from build123d import *

# Parameters (mm, degrees)
F0_R           = 90
F3_DEPTH       = 10
F4_D           = 5.5
F4_DEPTH       = 30
F4_TIP         = 1.6523667023
F6_D           = 3.6
F6_CBORE_D     = 6.6
F6_CBORE_DEPTH = 4
F8_D           = 3.6
F8_DEPTH       = 30
F8_TIP         = 1.0815491142
F9_DEPTH       = 5


with BuildPart() as f3:
    # F0 (on Top) → F3 (new body)
    with BuildSketch(Plane.XY):
        Circle(F0_R)
    extrude(amount=F3_DEPTH)

    # F4
    with Locations(Plane(origin=(0, 0, 0), x_dir=(1, 0, 0), z_dir=(0, 0, -1))):
        with Locations((32.5, -56.291651246), (32.5, 56.291651246), (-65, 0), (0, 0)):
            Hole(F4_D / 2, depth=F4_DEPTH)
            with Locations((0, 0, -(F4_DEPTH + F4_TIP / 2))):  # 118° drill point
                Cone(0, F4_D / 2, F4_TIP, mode=Mode.SUBTRACT)

    # F6 (through all)
    with Locations(Plane(origin=(0, 0, 0), x_dir=(1, 0, 0), z_dir=(0, 0, -1))):
        with Locations((14.0151126623, 15.35), (58.0151126623, 15.35), (14.0151126623, -15.35), (58.0151126623, -15.35)):
            CounterBoreHole(F6_D / 2, F6_CBORE_D / 2, F6_CBORE_DEPTH)

    # F8
    with Locations(Plane(origin=(0, 0, 0), x_dir=(1, 0, 0), z_dir=(0, 0, -1))):
        with Locations((-12.8155729771, 59.4439784884), (-20.8155729771, 59.4439784884), (-12.8155729771, 35.4439784884), (-20.8155729771, 35.4439784884), (-49.032068802, -39.4834254403), (-29.032068802, -39.4834254403), (-6.8313475791, -59.4414137304), (8.1686524209, -59.4414137304), (-23.532068802, 0.5165745633), (-54.532068802, 0.5165745597)):
            Hole(F8_D / 2, depth=F8_DEPTH)
            with Locations((0, 0, -(F8_DEPTH + F8_TIP / 2))):  # 118° drill point
                Cone(0, F8_D / 2, F8_TIP, mode=Mode.SUBTRACT)

    # F7 (on face) → F9 (cut)
    with BuildSketch(Plane.XY):
        with BuildLine():
            Line((-54.4565801894, 1.4820002999), (-54.6077416208, 1.4819933337))
            ThreePointArc((-54.6077416208, 1.4819933337), (-56.5317107433, -0.5544177441), (-54.532068802, -2.5165745597))
            ThreePointArc((-54.532068802, -2.5165745597), (-53.1178552397, -1.9307881221), (-52.532068802, -0.5165745597))
            ThreePointArc((-52.532068802, -0.5165745597), (-53.091413183, 0.8706930379), (-54.4565801894, 1.4820002999))
        make_face()
        with BuildLine():
            ThreePointArc((-23.5321609709, 1.4834254345), (-25.5320688015, -0.5166206477), (-23.5320688023, -2.5165745633))
            ThreePointArc((-23.5320688023, -2.5165745633), (-22.1178552398, -1.9307881258), (-21.532068802, -0.5165745633))
            ThreePointArc((-21.532068802, -0.5165745633), (-22.1178878267, 0.8976715853), (-23.5321609709, 1.4834254345))
        make_face()
        with BuildLine():
            ThreePointArc((-52.532068802, -0.5165745597), (-53.1178552397, -1.9307881221), (-54.532068802, -2.5165745597))
            Line((-54.532068802, -2.5165745597), (-23.5320688023, -2.5165745633))
            ThreePointArc((-23.5320688023, -2.5165745633), (-25.5320688015, -0.5166206477), (-23.5321609709, 1.4834254345))
            Line((-23.5321609709, 1.4834254345), (-54.4565801894, 1.4820002999))
            ThreePointArc((-54.4565801894, 1.4820002999), (-53.091413183, 0.8706930379), (-52.532068802, -0.5165745597))
        make_face()
        with BuildLine():
            ThreePointArc((-29.032068802, 37.4834254403), (-31.032068802, 39.4834254403), (-29.032068802, 41.4834254403))
            Line((-29.032068802, 41.4834254403), (-49.032068802, 41.4834254403))
            ThreePointArc((-49.032068802, 41.4834254403), (-47.6178552397, 40.8976390026), (-47.032068802, 39.4834254403))
            ThreePointArc((-47.032068802, 39.4834254403), (-47.6178552397, 38.0692118779), (-49.032068802, 37.4834254403))
            Line((-49.032068802, 37.4834254403), (-29.032068802, 37.4834254403))
        make_face()
        with BuildLine():
            ThreePointArc((-47.032068802, 39.4834254403), (-47.6178552397, 40.8976390026), (-49.032068802, 41.4834254403))
            ThreePointArc((-49.032068802, 41.4834254403), (-51.032068802, 39.4834254403), (-49.032068802, 37.4834254403))
            ThreePointArc((-49.032068802, 37.4834254403), (-47.6178552397, 38.0692118779), (-47.032068802, 39.4834254403))
        make_face()
        with BuildLine():
            ThreePointArc((-29.032068802, 37.4834254403), (-27.6178552397, 38.0692118779), (-27.032068802, 39.4834254403))
            ThreePointArc((-27.032068802, 39.4834254403), (-27.6178552397, 40.8976390026), (-29.032068802, 41.4834254403))
            ThreePointArc((-29.032068802, 41.4834254403), (-31.032068802, 39.4834254403), (-29.032068802, 37.4834254403))
        make_face()
        with BuildLine():
            ThreePointArc((-6.8313475791, 61.4414137304), (-5.4171340168, 60.8556272928), (-4.8313475791, 59.4414137304))
            ThreePointArc((-4.8313475791, 59.4414137304), (-5.4171340168, 58.027200168), (-6.8313475791, 57.4414137304))
            Line((-6.8313475791, 57.4414137304), (8.1686524209, 57.4414137304))
            ThreePointArc((8.1686524209, 57.4414137304), (6.1686524209, 59.4414137304), (8.1686524209, 61.4414137304))
            Line((8.1686524209, 61.4414137304), (-6.8313475791, 61.4414137304))
        make_face()
        with BuildLine():
            ThreePointArc((-6.8313475791, 57.4414137304), (-5.4171340168, 58.027200168), (-4.8313475791, 59.4414137304))
            ThreePointArc((-4.8313475791, 59.4414137304), (-5.4171340168, 60.8556272928), (-6.8313475791, 61.4414137304))
            ThreePointArc((-6.8313475791, 61.4414137304), (-8.8313475791, 59.4414137304), (-6.8313475791, 57.4414137304))
        make_face()
        with BuildLine():
            ThreePointArc((10.1686524209, 59.4414137304), (9.5828659832, 60.8556272928), (8.1686524209, 61.4414137304))
            ThreePointArc((8.1686524209, 61.4414137304), (6.1686524209, 59.4414137304), (8.1686524209, 57.4414137304))
            ThreePointArc((8.1686524209, 57.4414137304), (9.5828659832, 58.027200168), (10.1686524209, 59.4414137304))
        make_face()
    extrude(amount=F9_DEPTH, mode=Mode.SUBTRACT)


solid = f3.part
Here's how the part is built. I have some questions about the finished solid (model axes, mm). A direction names the side the tool comes from. Coordinates: 2 decimals unless noted, no trailing zeros. Write each loop counter-clockwise with the first axis right and the second up, starting at its lowest first coordinate (ties: lowest second). Pieces come first, ordered by that corner, then holes.
1) If we section it at C-C (x = 32.5): List the corners of the cut face in (y, z) for me.
Filled in:
outline: (-83.93, 0) - (-59.04, 0) - (-59.04, 10) - (-83.93, 10) - close; (-53.54, 0) - (53.54, 0) - (53.54, 10) - (-53.54, 10) - close; (59.04, 0) - (83.93, 0) - (83.93, 10) - (59.04, 10) - close
2) If I drill on line 1 (Y direction, x = 59, z = 6); line 2 (X direction, y = -15.35, z = 2.3); line 3 (Y direction, x = -32, z = 3.75), over which ranges is the centre line in solid material (lowest first)?
Filled in:
line 1: y = -67.96 to -16.86, -13.84 to 13.84, 16.86 to 67.96
line 2: x = -88.68 to 10.72, 17.32 to 54.72, 61.32 to 88.68
line 3: y = -84.12 to -2.52, 1.48 to 37.48, 41.48 to 84.12
3) I'm going to push flat-ended pins straight in: pin 1 (6 mm diameter, centred on x = 14.02, y = 15.35, fed in from -Z); pin 2 (4 mm diameter, centred on x = 33, z = 1, fed in from -Y); pin 3 (3 mm diameter, centred on x = 52.5, z = 1, fed in from -Y). Where does each tip first touch, or does it pass through?
Filled in:
pin 1: stops at z = 4
pin 2: stops at y = -84.49
pin 3: stops at y = -74.16
4) Thinking about a two-plate mould opening in Y: for faces 3 (the face through (19, 1, 10)), 4 (the face through (-39, 40, 5)), which applies, +Y half, -Y half, draft (parallel to the pull), parting line (faces both ways), or undercut?
Filled in:
face 3: draft
face 4: undercut
5) If we section it at A-A (x = 0): List the corners of the cut face in (y, z) for me, plus the area to 4 significant figures.
Filled in:
outline: (-90, 0) - (-2.75, 0) - (-2.75, 10) - (-90, 10) - close; (2.75, 0) - (57.44, 0) - (57.44, 5) - (61.44, 5) - (61.44, 0) - (90, 0) - (90, 10) - (2.75, 10) - close
area: 1,725 mm2
6) Which directions (+Z, -Z, +X, -X, +Y, -Y) give clear straight access to the entire face, cutting with the end or side of a thin tool? Please do faces 1 (the face through (19, 1, 0)), 2 (the face through (-8.83, 59.49, 2.46)).
Filled in:
face 1: -Z, +X, -X, +Y, -Y
face 2: -Z
7) If we section it at B-B (z = 2): Count the separate pieces of the cut face and the enclosed holes in it, plus the area to 3 significant figures.
Filled in:
separate pieces: 1
enclosed holes: 15
area: 24,900 mm2
8) If we section it at D-D (y = -42): List the corners of the cut face in (x, z) for me, plus the area to 3 significant figures.
Filled in:
outline: (-79.6, 0) - (79.6, 0) - (79.6, 10) - (-79.6, 10) - close
area: 1,590 mm2
